from build123d import *

# Parameters (mm, degrees)
F0_W     = 28.348149
F0_H     = 6.35
F0_W_2   = 6.35
F0_H_2   = 25.4
F0_R     = 48.895
F1_DEPTH = 6.35


with BuildPart() as f1:
    # F0 (on Front) → F1 (new body)
    with BuildSketch(Plane.XZ):
        Polygon((26.302561, 63.5), (-26.302561, 63.5), (-63.5, 26.302561), (-107.699501, 14.567526), (-107.699501, -14.531948), (-63.279638, -26.522923), (-26.302561, -63.5), (26.302561, -63.5), (63.279638, -26.522923), (107.699501, -14.531948), (107.699501, 14.567526), (63.5, 26.302561), align=None)
        with Locations((-75.024232, -9.525)):
            Rectangle(F0_W, F0_H, mode=Mode.SUBTRACT)
        with Locations((0, -56.1975)):
            Rectangle(F0_W_2, F0_H, mode=Mode.SUBTRACT)
        with Locations((75.024232, -9.525)):
            Rectangle(F0_W, F0_H, mode=Mode.SUBTRACT)
        with Locations((-97.453307, 0)):
            Rectangle(F0_W_2, F0_H_2, mode=Mode.SUBTRACT)
        with Locations((-75.024232, 9.525)):
            Rectangle(F0_W, F0_H, mode=Mode.SUBTRACT)
        Circle(F0_R, mode=Mode.SUBTRACT)
        with Locations((75.024232, 9.525)):
            Rectangle(F0_W, F0_H, mode=Mode.SUBTRACT)
        with Locations((97.453307, 0)):
            Rectangle(F0_W_2, F0_H_2, mode=Mode.SUBTRACT)
        with Locations((0, 56.1975)):
            Rectangle(F0_W_2, F0_H, mode=Mode.SUBTRACT)
    extrude(amount=F1_DEPTH)


solid = f1.part
CAD build for the part. Positions are in the model's coordinates, mm. A direction names the side the tool comes from. Round coordinates to 2 decimals unless told otherwise and drop trailing zeros. Write each loop counter-clockwise with the first axis right and the second up, starting at its lowest first coordinate (ties: lowest second). Pieces come first, ordered by that corner, then holes.
(1) Slice it at C-C, the plane z = 46. Write the cut outline in (x, y), and give its area (3 significant figures).
(2) Slice it at A-A, the plane x = 0. Count the separate pieces of the cut face and the enclosed holes in it, and give its area (3 significant figures).
(3) Drop flat-ended pins along their axis: P1, Ø12, axis at x = 43, z = 20, coming from the -Y side; P2, Ø1.9, axis at x = -75, y = -1.5, coming from the +Z side; P3, Ø1, axis at x = -64.5, y = -1, coming from the -Z side; P4, Ø3, axis at y = -1.5, z = 57, coming from the +X side. Give the stop position or say it passes through.
(4) 3-axis set-ups, long thin cutter, end or side, ignore diameter. For faces 4 (the face through (-45, -3.1, -44.8)), 5 (the face through (97, -3, -12.7)): which of +Z, -Z, +X, -X, +Y, -Y reach the whole face in a straight line?
(5) Mould opens along X. For faces 1 (the face through (44.5, -3.1, -45.3)), 2 (the face through (0, -3, 53.022)), 3 (the face through (0, -3, -63.5)) say: pulls with the +X half, pulls with the -X half, needs draft (parallel to the pull), parting line crosses it, or undercut.
(6) Probe line 1 along Z through (x, y) = (0, -4.25) (1 decimal); line 2 along Z through (x, y) = (-86, -5); line 3 along X through (y, z) = (-4.5, 53.5) (3 decimals). List the from-to ranges inside material, lowest first.
From the geometry:
1. outline: (-43.8, -6.35) - (-16.57, -6.35) - (-16.57, 0) - (-43.8, 0) - close; (16.57, -6.35) - (43.8, -6.35) - (43.8, 0) - (16.57, 0) - close
1. area: 346 mm2
2. separate pieces: 4
2. enclosed holes: 0
2. area: 105 mm2
3. P1: stops at y = -6.35
3. P2: stops at z = 23.5
3. P3: stops at z = -26.33
3. P4: stops at x = 34.3
4. face 4: -Z, -X, +Y, -Y
4. face 5: +Y, -Y
5. face 1: pulls with the +X half
5. face 2: undercut
5. face 3: needs draft
6. line 1: z = -63.5 to -59.4, -53 to -48.9, 48.9 to 53, 59.4 to 63.5
6. line 2: z = -20.39 to -12.7, -6.35 to 6.35, 12.7 to 20.33
6. line 3: x = -36.303 to -3.175, 3.175 to 36.303
